Geometry: final body of the model. Coordinates: model frame, mm. A direction names the side the tool comes from. Give positions to 0.01 mm unless a question says otherwise; leave off trailing zeros. Loops run counter-clockwise (first coordinate to the right, second up) from the corner with the lowest first, then second, coordinate; pieces in that order, holes last.
from build123d import *

# Parameters (mm, degrees)
F0_W     = 16
F0_H     = 16
F0_W_2   = 13
F0_H_2   = 13
F1_DEPTH = 16
F3_DEPTH = 6.3


with BuildPart() as f1:
    # F0 (on Top) → F1 (new body)
    with BuildSketch(Plane.XY):
        Rectangle(F0_W, F0_H)
        Rectangle(F0_W_2, F0_H_2, mode=Mode.SUBTRACT)
    extrude(amount=F1_DEPTH)

    # F2 (on Top) → F3 (join)
    with BuildSketch(Plane.XY):
        Polygon((-18.4455, 20), (-18.4455, -20), (21.5545, -20), (21.5545, 20), (0, 20), align=None)
    extrude(amount=F3_DEPTH)


solid = f1.part
Item 1: Section query B-B on x = 0. Return loops of the section in (y, z).
Values follow:
outline: (-20, 0) - (20, 0) - (20, 6.3) - (8, 6.3) - (8, 16) - (6.5, 16) - (6.5, 6.3) - (-6.5, 6.3) - (-6.5, 16) - (-8, 16) - (-8, 6.3) - (-20, 6.3) - close
Item 2: Section query C-C on y = 7. Return loops of the section in (x, z), plus the area to 3 significant figures.
Values follow:
outline: (-18.45, 0) - (21.55, 0) - (21.55, 6.3) - (8, 6.3) - (8, 16) - (-8, 16) - (-8, 6.3) - (-18.45, 6.3) - close
area: 407 mm2
Item 3: Ray query, probe 1 along Y at (x, z) = (1, 11.75); probe 2 along Z at (x, y) = (18, 4.5). Return the intervals inside material, ascending.
Values follow:
probe 1: y = -8 to -6.5, 6.5 to 8
probe 2: z = 0 to 6.3
Item 4: Set-up query: faces 1 (the face through (0, -6.5, 11)), 2 (the face through (8, 0, 11)), 3 (the face through (0, 8, 11)). Return all of +Z, -Z, +X, -X, +Y, -Y with unobstructed straight access to the full face (end or side cutting, diameter ignored); none if empty.
Values follow:
face 1: +Z
face 2: +Z, +X, +Y, -Y
face 3: +Z, +X, -X, +Y
Item 5: Section query D-D on x = -7. Return loops of the section in (y, z), plus the area to 3 significant figures.
Values follow:
outline: (-20, 0) - (20, 0) - (20, 6.3) - (8, 6.3) - (8, 16) - (-8, 16) - (-8, 6.3) - (-20, 6.3) - close
area: 407 mm2
Item 6: Section query A-A on z = 14. Return loops of the section in (x, y).
Values follow:
outline: (-8, -8) - (8, -8) - (8, 8) - (-8, 8) - close; hole (-6.5, -6.5) - (6.5, -6.5) - (6.5, 6.5) - (-6.5, 6.5) - close
Item 7: Pin query (flat end, axial travel): pin 1 (10.5 mm diameter, centred on x = 1, y = -1, fed in from +Z); pin 2 (3 mm diameter, centred on x = 14.5, z = 8.5, fed in from +Y); pin 3 (5 mm diameter, centred on y = -1.5, z = 11.5, fed in from +X); pin 4 (3 mm diameter, centred on x = 3, z = 11, fed in from -Y). Return the tip coordinate at first contact, or that it passes through.
Values follow:
pin 1: stops at z = 6.3
pin 2: passes through
pin 3: stops at x = 8
pin 4: stops at y = -8
